The listing builds one solid part. Answer for the finished solid, in the listing's coordinates (mm). Face numbers are marked on the shaded views. A direction names the side the tool comes from. Round coordinates to 2 decimals unless told otherwise and drop trailing zeros. Order: outer loops, then holes, each group sorted by start corner. A loop starts at its lowest first (then second) coordinate and runs counter-clockwise, first axis right, second up. Notation, with made-up numbers: M 80.5,73.5 L 95.5,73.5 A26 ccw 95.5,88.5 Z; hole C 15,-36 d5. An arc over 180 degrees is marked long. Write item = value, one per line. Start each with the question number.
(1) For a pull along Z with two mould halves and no side action, classify the marked faces 3, 4 and 5 as released by +Z, released by -Z, zero draft, split by the parting line, or undercut.
(2) A cutting plane is placed at A-A, the plane y = -17. Determine the outline of the cut face in (x, z), and give its area (3 significant figures).
(3) Straight lines are drawn through the part: probe 1 along X at (y, z) = (-7, -46.5); probe 2 along X at (y, z) = (-15, -28); probe 3 along Z at (x, y) = (40, -15.5). For each, find the intervals that lie inside material, in ascending order. Write a range as from..to.
(4) Each of these flat-tipped pins is pushed along its axis until it touches: pin 1 (17.5 mm diameter, centred on x = 21, z = -44.5, fed in from -Y); pin 2 (1.5 mm diameter, centred on x = 38.5, y = -3, fed in from -Z); pin 3 (0.6 mm diameter, centred on x = 25.5, y = -0.5, fed in from +Z). Where does it stop, or does it pass through?
(5) A cutting plane is placed at D-D, the plane y = -10.5. Determine the outline of the cut face in (x, z).
(6) A cutting plane is placed at B-B, the plane x = 45. Determine the outline of the cut face in (y, z), and give its area (3 significant figures).
(7) A cutting plane is placed at C-C, the plane z = -18. Determine the outline of the cut face in (x, y).
(8) Which of the six approach directions +Z, -Z, +X, -X, +Y, -Y give full straight-line access (tool end or side, diameter ignored) to the marked faces 1 and 2?
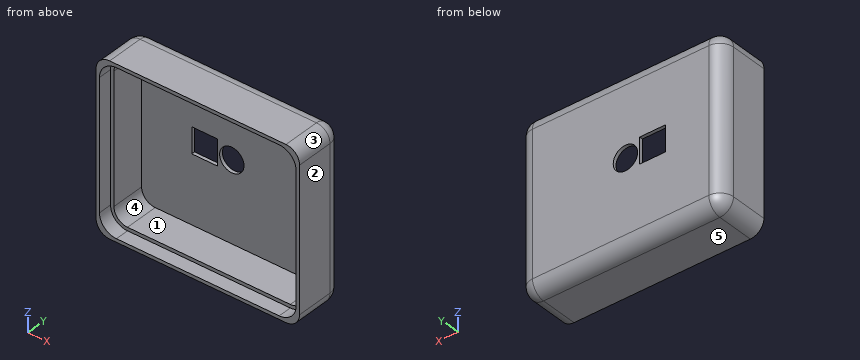
from build123d import *

# Parameters (mm, degrees)
BOSS_EXTRUDE1_DEPTH      = 0.000254
BOSS_EXTRUDE1_DEPTH_BACK = 19.05
SKETCH2_W                = 76.2
SKETCH2_H                = 63.5
SKETCH3_W                = 71.12
SKETCH3_H                = 58.42
CUT_EXTRUDE2_DEPTH       = 17.78
CUT_EXTRUDE3_DEPTH       = 2.54
CUT_EXTRUDE3_DEPTH_BACK  = 102.002933126
SKETCH2_3_R              = 4.572
SKETCH2_3_W              = 9.652
SKETCH2_3_H              = 9.652
FILLET1_R                = 5.08
FILLET2_R                = 5.08
FILLET3_R                = 5.08
FILLET4_R                = 5.08
FILLET5_R                = 5.08
FILLET6_R                = 5.08
CUT_EXTRUDE4_DEPTH       = 5.08


with BuildPart() as part:
    # Sketch2 → Boss-Extrude1 (new, two sides: drawn at the far end of the back side and taken through both)
    with BuildSketch(Plane(origin=(0, 0, 0), x_dir=(1, 0, 0), z_dir=(0, 1, 0)).offset(-BOSS_EXTRUDE1_DEPTH_BACK)):
        with Locations((38.1, 31.75)):
            Rectangle(SKETCH2_W, SKETCH2_H)
    extrude(amount=BOSS_EXTRUDE1_DEPTH + BOSS_EXTRUDE1_DEPTH_BACK)

    # Sketch3 → Cut-Extrude2 (cut)
    with BuildSketch(Plane(origin=(0, -19.05, 0), x_dir=(-1, 0, 0), z_dir=(0, -1, 0))):
        with Locations((-38.1, 31.75)):
            Rectangle(SKETCH3_W, SKETCH3_H)
    extrude(amount=-CUT_EXTRUDE2_DEPTH, mode=Mode.SUBTRACT)

    # Sketch2_3 → Cut-Extrude3 (cut, two sides: drawn at the far end of the back side and taken through both)
    with BuildSketch(Plane(origin=(0, 0, 0), x_dir=(1, 0, 0), z_dir=(0, 1, 0)).offset(-CUT_EXTRUDE3_DEPTH_BACK)):
        with Locations(Location((36.322, 31.064, 0), (0, 0, 90))):
            Circle(SKETCH2_3_R)
        with Locations((26.162, 30.81)):
            Rectangle(SKETCH2_3_W, SKETCH2_3_H)
    extrude(amount=CUT_EXTRUDE3_DEPTH + CUT_EXTRUDE3_DEPTH_BACK, mode=Mode.SUBTRACT)

    # Fillet1
    fillet1_edges = [part.edges().sort_by_distance(p)[0] for p in [
        (76.2, -9.524873, -63.5),
    ]]
    fillet(fillet1_edges, radius=FILLET1_R)

    # Fillet2
    fillet2_edges = [part.edges().sort_by_distance(p)[0] for p in [
        (73.66, -10.16, -60.96),
    ]]
    fillet(fillet2_edges, radius=FILLET2_R)

    # Fillet3
    fillet3_edges = [part.edges().sort_by_distance(p)[0] for p in [
        (73.66, -10.16, -2.54),
        (76.2, -9.524873, 0),
    ]]
    fillet(fillet3_edges, radius=FILLET3_R)

    # Fillet4
    fillet4_edges = [part.edges().sort_by_distance(p)[0] for p in [
        (2.54, -10.16, -2.54),
        (0, -9.524873, 0),
    ]]
    fillet(fillet4_edges, radius=FILLET4_R)

    # Fillet5
    fillet5_edges = [part.edges().sort_by_distance(p)[0] for p in [
        (2.54, -10.16, -60.96),
        (0, -9.524873, -63.5),
    ]]
    fillet(fillet5_edges, radius=FILLET5_R)

    # Fillet6
    fillet6_edges = [part.edges().sort_by_distance(p)[0] for p in [
        (38.1, 0.000254, -63.5),
        (1.487897552, 0.000254, -62.012102448),
        (74.712102448, 0.000254, -62.012102448),
        (76.2, 0.000254, -31.75),
        (74.712102448, 0.000254, -1.487897552),
        (0, 0.000254, -31.75),
        (38.1, 0.000254, 0),
        (1.487897552, 0.000254, -1.487897552),
    ]]
    fillet(fillet6_edges, radius=FILLET6_R)

    # Sketch5 → Cut-Extrude4 (cut)
    with BuildSketch(Plane.XZ.offset(19.05)):
        with BuildLine():
            Line((1.27, -7.62), (1.27, -55.88))
            ThreePointArc((1.27, -55.88), (3.129871939, -60.370128061), (7.62, -62.23))
            Line((7.62, -62.23), (68.58, -62.23))
            ThreePointArc((68.58, -62.23), (73.070128061, -60.370128061), (74.93, -55.88))
            Line((74.93, -55.88), (74.93, -7.62))
            ThreePointArc((74.93, -7.62), (73.070128061, -3.129871939), (68.58, -1.27))
            Line((68.58, -1.27), (7.62, -1.27))
            ThreePointArc((7.62, -1.27), (3.129871939, -3.129871939), (1.27, -7.62))
        make_face()
    extrude(amount=-CUT_EXTRUDE4_DEPTH, mode=Mode.SUBTRACT)


solid = part.part
Reported:
q1.face_3 = released by +Z
q1.face_4 = undercut
q1.face_5 = released by -Z
q2.outline = M 0,-58.42 A5.08 ccw 5.08,-63.5 L 71.12,-63.5 A5.08 ccw 76.2,-58.42 L 76.2,-5.08 A5.08 ccw 71.12,0 L 5.08,0 A5.08 ccw 0,-5.08 Z; hole M 1.27,-55.88 A6.35 ccw 7.62,-62.23 L 68.58,-62.23 A6.35 ccw 74.93,-55.88 L 74.93,-7.62 A6.35 ccw 68.58,-1.27 L 7.62,-1.27 A6.35 ccw 1.27,-7.62 Z
q2.area = 361 mm²
q3.probe_1 = 0..2.54, 73.66..76.2
q3.probe_2 = 0..1.27, 74.93..76.2
q3.probe_3 = -63.5..-62.23, -1.27..0
q4.pin_1 = -1.27
q4.pin_2 = -63.32
q4.pin_3 = -2.34
q5.outline = M 0,-58.42 A5.08 ccw 5.08,-63.5 L 71.12,-63.5 A5.08 ccw 76.2,-58.42 L 76.2,-5.08 A5.08 ccw 71.12,0 L 5.08,0 A5.08 ccw 0,-5.08 Z; hole M 2.54,-55.88 A5.08 ccw 7.62,-60.96 L 68.58,-60.96 A5.08 ccw 73.66,-55.88 L 73.66,-7.62 A5.08 ccw 68.58,-2.54 L 7.62,-2.54 A5.08 ccw 2.54,-7.62 Z
q6.outline = M -19.05,-63.5 L -5.08,-63.5 A5.08 ccw 0,-58.42 L 0,-5.08 A5.08 ccw -5.08,0 L -19.05,0 L -19.05,-1.27 L -13.97,-1.27 L -13.97,-2.54 L -1.27,-2.54 L -1.27,-60.96 L -13.97,-60.96 L -13.97,-62.23 L -19.05,-62.23 Z
q6.area = 147 mm²
q7.outline = M 0,-19.05 L 1.27,-19.05 L 1.27,-13.97 L 2.54,-13.97 L 2.54,-1.27 L 73.66,-1.27 L 73.66,-13.97 L 74.93,-13.97 L 74.93,-19.05 L 76.2,-19.05 L 76.2,-5.08 A5.08 ccw 71.12,0 L 5.08,0 A5.08 ccw 0,-5.08 Z
q8.face_1 = -Y
q8.face_2 = +Z, -Z, +X, +Y, -Y
